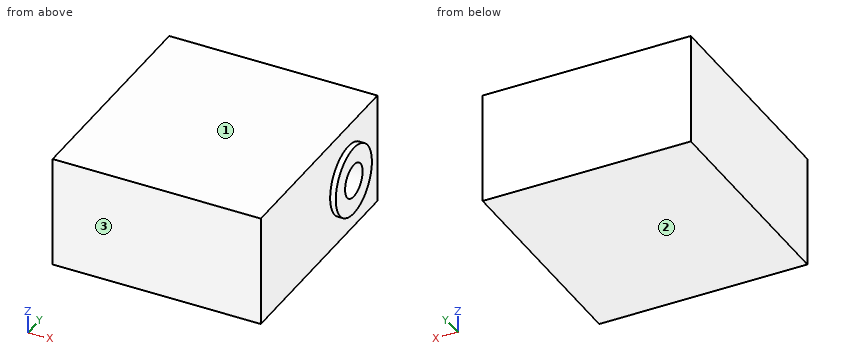
```python
from build123d import *

# Parameters (mm, degrees)
SKETCH1_W           = 37.2
SKETCH1_H           = 20
BOSS_EXTRUDE1_DEPTH = 40
SKETCH2_R           = 6.2
BOSS_EXTRUDE2_DEPTH = 1
SKETCH3_R           = 3
CUT_EXTRUDE1_DEPTH  = 10


with BuildPart() as part:
    # Sketch1 → Boss-Extrude1 (new body)
    with BuildSketch(Plane(origin=(0, 0, 0), x_dir=(1, 0, 0), z_dir=(0, 1, 0))):
        with Locations((-18.6, 10)):
            Rectangle(SKETCH1_W, SKETCH1_H)
    extrude(amount=BOSS_EXTRUDE1_DEPTH)

    # Sketch2 → Boss-Extrude2 (add)
    with BuildSketch(Plane(origin=(0, 0, 0), x_dir=(0, 0, -1), z_dir=(1, 0, 0))):
        with Locations(Location((10, 30, 0), (0, 0, 180))):
            Circle(SKETCH2_R)
    extrude(amount=BOSS_EXTRUDE2_DEPTH)

    # Sketch3 → Cut-Extrude1 (cut)
    with BuildSketch(Plane(origin=(1, 0, 0), x_dir=(0, 0, -1), z_dir=(1, 0, 0))):
        with Locations((10, 30)):
            Circle(SKETCH3_R)
    extrude(amount=-CUT_EXTRUDE1_DEPTH, mode=Mode.SUBTRACT)


solid = part.part
```
Here's how the part is built. I have some questions about the finished solid (model axes, mm). Face numbers are marked on the shaded views. Coordinates: 2 decimals unless noted, no trailing zeros. Order: outer loops, then holes, each group sorted by start corner. A loop starts at its lowest first (then second) coordinate and runs counter-clockwise, first axis right, second up.
Item 1: If we section it at D-D, the plane z = -5: List the corners of the cut face in (x, y) for me, then the cut area to 3 significant figures.
Response values:
outline: (-37.2, 0) - (0, 0) - (0, 26.33) - (1, 26.33) - (1, 33.67) - (0, 33.67) - (0, 40) - (-37.2, 40) - close
area: 1,500 mm2
Item 2: I need wall thicknesses on probe 1 along Y at (x, z) = (-2, -10); probe 2 along X at (y, z) = (17, -8.5); probe 3 along X at (y, z) = (31, -8). Which ranges of each line are inside material? Lowest first, please.
Response values:
probe 1: y = 0 to 27, 33 to 40
probe 2: x = -37.2 to 0
probe 3: x = -37.2 to -9
Item 3: If we section it at B-B, the plane z = -10: List the corners of the cut face in (x, y) for me.
Response values:
outline: (-37.2, 0) - (0, 0) - (0, 23.8) - (1, 23.8) - (1, 27) - (-9, 27) - (-9, 33) - (1, 33) - (1, 36.2) - (0, 36.2) - (0, 40) - (-37.2, 40) - close
Item 4: If we section it at A-A, the plane x = -4.5: List the corners of the cut face in (y, z) for me, then the cut area to 3 significant figures.
Response values:
outline: (0, -20) - (40, -20) - (40, 0) - (0, 0) - close; hole circle Ø6 at (30, -10)
area: 772 mm2
Item 5: I'm going to push flat-ended pins straight in: pin 1 Ø4 at (y, z) = (13, -17.5) entering from +X; pin 2 Ø3.5 at (y, z) = (30, -10) entering from +X. Where does each tip first touch, or does it pass through?
Response values:
pin 1: stops at x = 0
pin 2: stops at x = -9
Item 6: Thinking about a two-plate mould opening in Z: for the marked faces 1, 2 and 3, which applies, pulls with the +Z half, pulls with the -Z half, needs draft (parallel to the pull), parting line crosses it, or undercut?
Response values:
face 1: pulls with the +Z half
face 2: pulls with the -Z half
face 3: needs draft
Item 7: If we section it at C-C, the plane y = 30: List the corners of the cut face in (x, z) for me.
Response values:
outline: (-37.2, -20) - (0, -20) - (0, -16.2) - (1, -16.2) - (1, -13) - (-9, -13) - (-9, -7) - (1, -7) - (1, -3.8) - (0, -3.8) - (0, 0) - (-37.2, 0) - close
